Can you work these out from the model? Positions are in its coordinate system, mm. A direction names the side the tool comes from. Round coordinates to 2 decimals unless told otherwise and drop trailing zeros. Write each loop counter-clockwise with the first axis right and the second up, starting at its lowest first coordinate (ties: lowest second). Pieces come first, ordered by that corner, then holes. Notation, with made-up numbers: (80, 61.5) - (135, 61.5) arc R34 ccw to (135, 96.5) - close; hole circle Ø11 at (71.5, -29.5). An arc over 180 degrees is marked (long way). One line per item, written item: value. Start each with the question number.
(1) Thinking about a two-plate mould opening in Y: for faces 1 (the face through (29.95, -28, -23)), 2 (the face through (-3.12, 4.7, -23.02)), 3 (the face through (16.9, 0.09, -23.08)), which applies, +Y half, -Y half, draft (parallel to the pull), parting line (faces both ways), or undercut?
(2) On a 3-axis mill with a long thin cutter (end or side, diameter ignored), from which of +Z, -Z, +X, -X, +Y, -Y can I reach the whole of each face in a straight line? I mean faces 4 (the face through (-0.1, -32, -23)), 5 (the face through (-4.55, -28, -23)). Say none if no direction works.
(3) I want a section at C-C on x = 23.5. List the corners of the cut face in (y, z) for me, plus the area to 3 significant figures.
(4) I want a section at A-A on y = -13. List the corners of the cut face in (x, z) for me.
(5) I'm going to push a flat-ended pin straight in: pin 1 Ø6 at (x, y) = (12.5, -52) entering from -Z. Where does the tip first touch, or does it pass through?
(6) I want a section at B-B on z = -22.8. List the corners of the cut face in (x, y) for me.
(7) If I drill on L1, parallel to Y at x = 6.35, z = -23.9; L2, parallel to X at y = -45, z = -24.65; L3, parallel to Y at x = 8, z = -23.7, over which ranges is the centre line in solid material (lowest first)? Write a range as from..to.
(8) I want a section at D-D on y = 0. List the corners of the cut face in (x, z) for me, plus the area to 3 significant figures.
from build123d import *

# Parameters (mm, degrees)
SKETCH3_W           = 34.5
SKETCH3_H           = 67.853
SKETCH3_R           = 2.15
SKETCH3_W_2         = 25.6
SKETCH3_H_2         = 50.75
BOSS_EXTRUDE1_DEPTH = 4.45
FILLET1_R           = 5


with BuildPart() as part:
    # Sketch3 → Boss-Extrude1 (new body)
    with BuildSketch(Plane.XY.offset(-25.278270569)):
        with Locations((12.7, -27.7265)):
            Rectangle(SKETCH3_W, SKETCH3_H)
        with Locations((6.35, 0)):
            Circle(SKETCH3_R, mode=Mode.SUBTRACT)
        with Locations((19.05, 0)):
            Circle(SKETCH3_R, mode=Mode.SUBTRACT)
        with Locations((12.7, -31.828)):
            Rectangle(SKETCH3_W_2, SKETCH3_H_2, mode=Mode.SUBTRACT)
    extrude(amount=BOSS_EXTRUDE1_DEPTH)

    # Fillet1
    fillet1_edges = [part.edges().sort_by_distance(p)[0] for p in [
        (29.95, -61.653, -23.053270569),
        (-4.55, -61.653, -23.053270569),
        (-4.55, 6.2, -23.053270569),
        (29.95, 6.2, -23.053270569),
    ]]
    fillet(fillet1_edges, radius=FILLET1_R)


solid = part.part
Established:
1. face 1: draft
1. face 2: +Y half
1. face 3: undercut
2. face 4: +Z, -Z
2. face 5: +Z, -Z, -X, +Y, -Y
3. outline: (-61.65, -25.28) - (-57.2, -25.28) - (-57.2, -20.83) - (-61.65, -20.83) - close; (-6.45, -25.28) - (6.2, -25.28) - (6.2, -20.83) - (-6.45, -20.83) - close
3. area: 76.1 mm2
4. outline: (-4.55, -25.28) - (-0.1, -25.28) - (-0.1, -20.83) - (-4.55, -20.83) - close; (25.5, -25.28) - (29.95, -25.28) - (29.95, -20.83) - (25.5, -20.83) - close
5. pin 1: through
6. outline: (-4.55, -56.65) arc R5 ccw to (0.45, -61.65) - (24.95, -61.65) arc R5 ccw to (29.95, -56.65) - (29.95, 1.2) arc R5 ccw to (24.95, 6.2) - (0.45, 6.2) arc R5 ccw to (-4.55, 1.2) - close; hole (-0.1, -57.2) - (25.5, -57.2) - (25.5, -6.45) - (-0.1, -6.45) - close; hole circle Ø4.3 at (6.35, 0); hole circle Ø4.3 at (19.05, 0)
7. L1: -61.65..-57.2, -6.45..-2.15, 2.15..6.2
7. L2: -4.55..-0.1, 25.5..29.95
7. L3: -61.65..-57.2, -6.45..-1.38, 1.38..6.2
8. outline: (-4.55, -25.28) - (4.2, -25.28) - (4.2, -20.83) - (-4.55, -20.83) - close; (8.5, -25.28) - (16.9, -25.28) - (16.9, -20.83) - (8.5, -20.83) - close; (21.2, -25.28) - (29.95, -25.28) - (29.95, -20.83) - (21.2, -20.83) - close
8. area: 115 mm2
